Design review of the part built by this model. Coordinates are the model's own, in mm. Face numbers are marked on the shaded views. Give positions to 0.01 mm unless a question says otherwise; leave off trailing zeros. Order: outer loops, then holes, each group sorted by start corner. A loop starts at its lowest first (then second) coordinate and runs counter-clockwise, first axis right, second up. Notation, with made-up numbers: (-1, 0.25) -> (58, 0.25) arc R33 ccw to (58, 32.25) -> close; hole circle Ø9 at (13, 59.5). An arc over 180 degrees is marked (long way). One line per item, written item: value.
from build123d import *

# Parameters (mm, degrees)
PAD_DEPTH    = 45.5
SKETCH001_R  = 1.4
POCKET_DEPTH = 6


with BuildPart() as part:
    # Sketch → Pad (new body)
    with BuildSketch(Plane.XY):
        with BuildLine():
            Line((12.715, 0), (12.715, 10))
            Line((12.715, 10), (-12.715, 10))
            Line((-12.715, 10), (-12.715, 0))
            Line((-12.715, 0), (-4.390988, 0))
            Line((-2.984796, 1.799844), (-4.390988, 0))
            ThreePointArc((-2.984796, 1.799844), (-2.906077, 2.115568), (-3.088032, 2.385328))
            Line((-5.817952, 4.091171), (-3.088032, 2.385328))
            ThreePointArc((-5.5, 5.2), (-6.076757, 4.765382), (-5.817952, 4.091171))
            Line((-5.5, 5.2), (5.5, 5.2))
            ThreePointArc((5.817952, 4.091171), (6.076757, 4.765382), (5.5, 5.2))
            Line((5.817952, 4.091171), (3.088032, 2.385328))
            ThreePointArc((3.088032, 2.385328), (2.906077, 2.115568), (2.984796, 1.799844))
            Line((2.984796, 1.799844), (4.390988, 0))
            Line((4.390988, 0), (12.715, 0))
        make_face()
    extrude(amount=PAD_DEPTH)

    # Sketch001 (on Face6 of Pad) → Pocket (cut)
    with BuildSketch(Plane(origin=(0, 10, 0), x_dir=(-1, 0, 0), z_dir=(0, 1, 0))):
        with Locations((-10, 12)):
            Circle(SKETCH001_R)
        with Locations((-10, 32)):
            Circle(SKETCH001_R)
        with Locations((10, 32)):
            Circle(SKETCH001_R)
        with Locations((10, 12)):
            Circle(SKETCH001_R)
    extrude(amount=-POCKET_DEPTH, mode=Mode.SUBTRACT)


solid = part.part
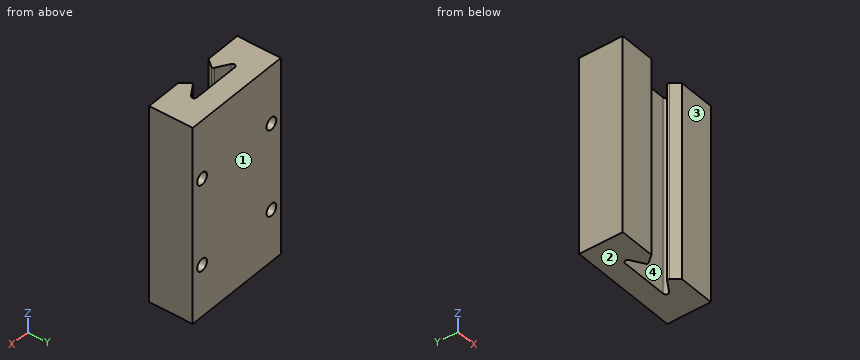
Item 1: Clearance check with flat-ended pins moving along their axes: P1, Ø5.5, axis at x = -1, z = 31.5, coming from the -Y side; P2, Ø1.4, axis at x = -9.5, z = 12, coming from the +Y side. State where each tip first meets the part, or that it passes through.
Returned:
P1: y = 0.82
P2: y = 4
Item 2: Add section A-A on y = 7.25. Give the boundary of the cut face in (x, z) (3 decimals), plus the area to 3 significant figures.
Returned:
outline: (-12.715, 0) -> (12.715, 0) -> (12.715, 45.5) -> (-12.715, 45.5) -> close; hole circle Ø2.8 at (-10, 12); hole circle Ø2.8 at (-10, 32); hole circle Ø2.8 at (10, 12); hole circle Ø2.8 at (10, 32)
area: 1,130 mm²
Item 3: Draft analysis for pull direction Y (two halves, no side actions). For the marked faces 1, 2, 3 and 4, state which applies: pulls with the +Y half, pulls with the -Y half, needs draft (parallel to the pull), parting line crosses it, or undercut.
Returned:
face 1: pulls with the +Y half
face 2: needs draft
face 3: pulls with the -Y half
face 4: undercut
Item 4: To check wall thickness, follow line 1 along Z through (x, y) = (-10, 8.8); line 2 along Y through (x, z) = (-2.5, 21.5); line 3 along Y through (x, z) = (-10.75, 11.5). State the ranges of each line that lie inside material, in increasing order. Write a range as from..to.
Returned:
line 1: 0..10.6, 13.4..30.6, 33.4..45.5
line 2: 5.2..10
line 3: 0..4
Item 5: Add section D-D on z = 21. Give the boundary of the cut face in (x, y) (3 decimals), plus the area to 3 significant figures.
Returned:
outline: (-12.715, 0) -> (-4.391, 0) -> (-2.985, 1.8) arc R0.4 ccw to (-3.088, 2.385) -> (-5.818, 4.091) arc R0.6 cw to (-5.5, 5.2) -> (5.5, 5.2) arc R0.6 cw to (5.818, 4.091) -> (3.088, 2.385) arc R0.4 ccw to (2.985, 1.8) -> (4.391, 0) -> (12.715, 0) -> (12.715, 10) -> (-12.715, 10) -> close
area: 209 mm²
Item 6: Add section B-B on z = 12. Give the boundary of the cut face in (x, y) (3 decimals).
Returned:
outline: (-12.715, 0) -> (-4.391, 0) -> (-2.985, 1.8) arc R0.4 ccw to (-3.088, 2.385) -> (-5.818, 4.091) arc R0.6 cw to (-5.5, 5.2) -> (5.5, 5.2) arc R0.6 cw to (5.818, 4.091) -> (3.088, 2.385) arc R0.4 ccw to (2.985, 1.8) -> (4.391, 0) -> (12.715, 0) -> (12.715, 10) -> (11.4, 10) -> (11.4, 4) -> (8.6, 4) -> (8.6, 10) -> (-8.6, 10) -> (-8.6, 4) -> (-11.4, 4) -> (-11.4, 10) -> (-12.715, 10) -> close
Item 7: Add section C-C on x = -10. Give the boundary of the cut face in (y, z), plus the area to 3 significant figures.
Returned:
outline: (0, 0) -> (10, 0) -> (10, 10.6) -> (4, 10.6) -> (4, 13.4) -> (10, 13.4) -> (10, 30.6) -> (4, 30.6) -> (4, 33.4) -> (10, 33.4) -> (10, 45.5) -> (0, 45.5) -> close
area: 421 mm²
